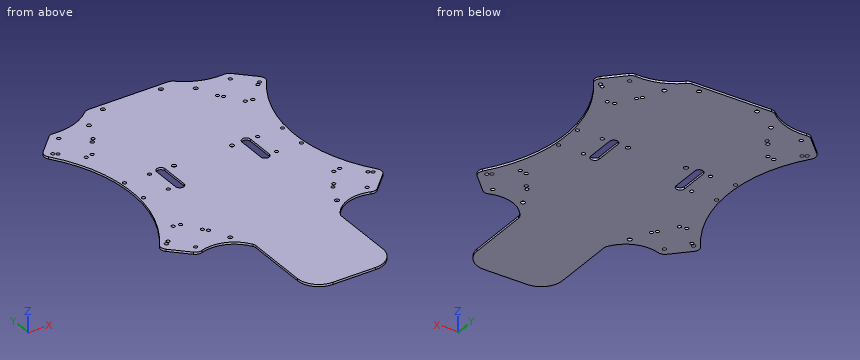
from build123d import *

# Parameters (mm, degrees)
SKETCH2_R           = 1.5
SKETCH2_R_2         = 1.25
BOSS_EXTRUDE1_DEPTH = 1.5
SKETCH3_R           = 1.25
F_45_DEGREES_DEPTH  = 170.629743854
SKETCH4_R           = 1.5
ODROID_HOLES_DEPTH  = 170.629743854
FILLET1_R           = 5
FILLET2_R           = 5
FILLET3_R           = 5
FILLET4_R           = 5
FILLET5_R           = 5
FILLET6_R           = 5
FILLET7_R           = 5
FILLET8_R           = 5
FILLET9_R           = 5
FILLET10_R          = 5
FILLET11_R          = 5
FILLET12_R          = 5
SKETCH5_R           = 1.25
F_35_DEGREES_DEPTH  = 169.878448293


with BuildPart() as part:
    # Sketch2 → Boss-Extrude1 (new body)
    with BuildSketch(Plane.XY):
        with BuildLine():
            Line((-79.195959493, 62.225396744), (-62.225396744, 79.195959493))
            ThreePointArc((-62.225396744, 79.195959493), (-44.806778225, 80.702789346), (-30, 90))
            Line((-30, 90), (30, 90))
            ThreePointArc((30, 90), (44.806778225, 80.702789346), (62.225396744, 79.195959493))
            Line((62.225396744, 79.195959493), (79.195959493, 62.225396744))
            ThreePointArc((79.195959493, 62.225396744), (57.477502656, 0), (79.195959493, -62.225396744))
            Line((79.195959493, -62.225396744), (62.225396744, -79.195959493))
            ThreePointArc((62.225396744, -79.195959493), (43.875108319, -77.923881554), (30, -90))
            Line((30, -90), (30, -135))
            ThreePointArc((30, -135), (25.606601718, -145.606601718), (15, -150))
            Line((15, -150), (-15, -150))
            ThreePointArc((-15, -150), (-25.606601718, -145.606601718), (-30, -135))
            Line((-30, -135), (-30, -90))
            ThreePointArc((-30, -90), (-43.875108319, -77.923881554), (-62.225396744, -79.195959493))
            Line((-62.225396744, -79.195959493), (-79.195959493, -62.225396744))
            ThreePointArc((-79.195959493, -62.225396744), (-57.477502656, 0), (-79.195959493, 62.225396744))
        make_face()
        with Locations((-37.5, 75)):
            Circle(SKETCH2_R, mode=Mode.SUBTRACT)
        with Locations((37.5, 75)):
            Circle(SKETCH2_R, mode=Mode.SUBTRACT)
        with Locations((37.5, -75)):
            Circle(SKETCH2_R, mode=Mode.SUBTRACT)
        with Locations((-37.5, -75)):
            Circle(SKETCH2_R, mode=Mode.SUBTRACT)
        with Locations((-55.5, 10)):
            Circle(SKETCH2_R_2, mode=Mode.SUBTRACT)
        with Locations((-38, 10)):
            Circle(SKETCH2_R_2, mode=Mode.SUBTRACT)
        with Locations((-55.5, -10)):
            Circle(SKETCH2_R_2, mode=Mode.SUBTRACT)
        with Locations((-38, -10)):
            Circle(SKETCH2_R_2, mode=Mode.SUBTRACT)
        with Locations((55.5, -10)):
            Circle(SKETCH2_R_2, mode=Mode.SUBTRACT)
        with Locations((38, -10)):
            Circle(SKETCH2_R_2, mode=Mode.SUBTRACT)
        with Locations((38, 10)):
            Circle(SKETCH2_R_2, mode=Mode.SUBTRACT)
        with Locations((55.5, 10)):
            Circle(SKETCH2_R_2, mode=Mode.SUBTRACT)
        with BuildLine():
            Line((27, -10), (27, 10))
            ThreePointArc((27, 10), (30, 13), (33, 10))
            Line((33, 10), (33, -10))
            ThreePointArc((33, -10), (30, -13), (27, -10))
        make_face(mode=Mode.SUBTRACT)
        with BuildLine():
            Line((-27, -10), (-27, 10))
            ThreePointArc((-27, 10), (-30, 13), (-33, 10))
            Line((-33, 10), (-33, -10))
            ThreePointArc((-33, -10), (-30, -13), (-27, -10))
        make_face(mode=Mode.SUBTRACT)
    extrude(amount=BOSS_EXTRUDE1_DEPTH)

    # Sketch3 → 45 Degrees (cut, through all)
    with BuildSketch(Plane.XY.offset(1.5)):
        with Locations((-72.655221767, 60.280853096)):
            Circle(SKETCH3_R)
        with Locations((-58.513086143, 46.138717472)):
            Circle(SKETCH3_R)
        with Locations(Location((-60.280853096, 72.655221767, 0), (0, 0, 180))):
            Circle(SKETCH3_R)
        with Locations(Location((-46.138717472, 58.513086143, 0), (0, 0, 180))):
            Circle(SKETCH3_R)
        with Locations(Location((58.513086143, 46.138717472, 0), (0, 0, 180))):
            Circle(SKETCH3_R)
        with Locations(Location((72.655221767, 60.280853096, 0), (0, 0, 180))):
            Circle(SKETCH3_R)
        with Locations((60.280853096, 72.655221767)):
            Circle(SKETCH3_R)
        with Locations((46.138717472, 58.513086143)):
            Circle(SKETCH3_R)
        with Locations(Location((-58.513086143, -46.138717472, 0), (0, 0, 180))):
            Circle(SKETCH3_R)
        with Locations((-46.138717472, -58.513086143)):
            Circle(SKETCH3_R)
        with Locations((-60.280853096, -72.655221767)):
            Circle(SKETCH3_R)
        with Locations(Location((-72.655221767, -60.280853096, 0), (0, 0, 180))):
            Circle(SKETCH3_R)
        with Locations((58.513086143, -46.138717472)):
            Circle(SKETCH3_R)
        with Locations((72.655221767, -60.280853096)):
            Circle(SKETCH3_R)
        with Locations(Location((60.280853096, -72.655221767, 0), (0, 0, 180))):
            Circle(SKETCH3_R)
        with Locations(Location((46.138717472, -58.513086143, 0), (0, 0, 180))):
            Circle(SKETCH3_R)
    extrude(amount=-F_45_DEGREES_DEPTH, mode=Mode.SUBTRACT)

    # Sketch4 → ODroid holes (cut, through all)
    with BuildSketch(Plane.XY.offset(1.5)):
        with Locations((-20.76, 10)):
            Circle(SKETCH4_R)
        with Locations((20, 10)):
            Circle(SKETCH4_R)
        with Locations((-20.76, 85.5)):
            Circle(SKETCH4_R)
        with Locations((20, 85.5)):
            Circle(SKETCH4_R)
    extrude(amount=-ODROID_HOLES_DEPTH, mode=Mode.SUBTRACT)

    # Fillet1
    fillet1_edges = [part.edges().sort_by_distance(p)[0] for p in [
        (-30, -90, 0.75),
    ]]
    fillet(fillet1_edges, radius=FILLET1_R)

    # Fillet2
    fillet2_edges = [part.edges().sort_by_distance(p)[0] for p in [
        (-62.225396744, -79.195959493, 0.75),
    ]]
    fillet(fillet2_edges, radius=FILLET2_R)

    # Fillet3
    fillet3_edges = [part.edges().sort_by_distance(p)[0] for p in [
        (30, -90, 0.75),
    ]]
    fillet(fillet3_edges, radius=FILLET3_R)

    # Fillet4
    fillet4_edges = [part.edges().sort_by_distance(p)[0] for p in [
        (62.225396744, -79.195959493, 0.75),
    ]]
    fillet(fillet4_edges, radius=FILLET4_R)

    # Fillet5
    fillet5_edges = [part.edges().sort_by_distance(p)[0] for p in [
        (79.195959493, -62.225396744, 0.75),
    ]]
    fillet(fillet5_edges, radius=FILLET5_R)

    # Fillet6
    fillet6_edges = [part.edges().sort_by_distance(p)[0] for p in [
        (-79.195959493, -62.225396744, 0.75),
    ]]
    fillet(fillet6_edges, radius=FILLET6_R)

    # Fillet7
    fillet7_edges = [part.edges().sort_by_distance(p)[0] for p in [
        (-79.195959493, 62.225396744, 0.75),
    ]]
    fillet(fillet7_edges, radius=FILLET7_R)

    # Fillet8
    fillet8_edges = [part.edges().sort_by_distance(p)[0] for p in [
        (-62.225396744, 79.195959493, 0.75),
    ]]
    fillet(fillet8_edges, radius=FILLET8_R)

    # Fillet9
    fillet9_edges = [part.edges().sort_by_distance(p)[0] for p in [
        (-30, 90, 0.75),
    ]]
    fillet(fillet9_edges, radius=FILLET9_R)

    # Fillet10
    fillet10_edges = [part.edges().sort_by_distance(p)[0] for p in [
        (30, 90, 0.75),
    ]]
    fillet(fillet10_edges, radius=FILLET10_R)

    # Fillet11
    fillet11_edges = [part.edges().sort_by_distance(p)[0] for p in [
        (62.225396744, 79.195959493, 0.75),
    ]]
    fillet(fillet11_edges, radius=FILLET11_R)

    # Fillet12
    fillet12_edges = [part.edges().sort_by_distance(p)[0] for p in [
        (79.195959493, 62.225396744, 0.75),
    ]]
    fillet(fillet12_edges, radius=FILLET12_R)

    # Sketch5 → 35 Degrees (cut, through all)
    with BuildSketch(Plane.XY.offset(1.5)):
        with Locations(Location((-60.280853096, 72.655221767, 0), (0, 0, 180))):
            Circle(SKETCH5_R)
        with Locations((-70.218840229, 58.462305252)):
            Circle(SKETCH5_R)
        with Locations((-53.835799344, 46.990776525)):
            Circle(SKETCH5_R)
        with Locations((-43.79882923, 61.326369694)):
            Circle(SKETCH5_R)
        with Locations((60.280853096, 72.655221767)):
            Circle(SKETCH5_R)
        with Locations(Location((43.79882923, 61.326369694, 0), (0, 0, 180))):
            Circle(SKETCH5_R)
        with Locations(Location((53.835799344, 46.990776525, 0), (0, 0, 180))):
            Circle(SKETCH5_R)
        with Locations(Location((70.218840229, 58.462305252, 0), (0, 0, 180))):
            Circle(SKETCH5_R)
        with Locations(Location((-70.218840229, -58.462305252, 0), (0, 0, 180))):
            Circle(SKETCH5_R)
        with Locations((-60.280853096, -72.655221767)):
            Circle(SKETCH5_R)
        with Locations(Location((-53.835799344, -46.990776525, 0), (0, 0, 180))):
            Circle(SKETCH5_R)
        with Locations(Location((-43.79882923, -61.326369694, 0), (0, 0, 180))):
            Circle(SKETCH5_R)
        with Locations((70.218840229, -58.462305252)):
            Circle(SKETCH5_R)
        with Locations(Location((60.280853096, -72.655221767, 0), (0, 0, 180))):
            Circle(SKETCH5_R)
        with Locations((43.79882923, -61.326369694)):
            Circle(SKETCH5_R)
        with Locations((53.835799344, -46.990776525)):
            Circle(SKETCH5_R)
    extrude(amount=-F_35_DEGREES_DEPTH, mode=Mode.SUBTRACT)


solid = part.part
Part model, mm, in its own coordinate system. Coordinates: 2 decimals unless noted, no trailing zeros. Loops run counter-clockwise (first coordinate to the right, second up) from the corner with the lowest first, then second, coordinate; pieces in that order, holes last. Notation, with made-up numbers: M 18.25,47 L 32.25,47 A16 ccw 32.25,65 Z; hole C 56.5,-29.5 d5. An arc over 180 degrees is marked long. Use a Markdown table: item, result. Add a question column.
Q1. Cut at B-B (z = 0.45). Give the number of separate pieces and of enclosed holes in the cut face, and give its area (3 significant figures).
Q2. Probe L1, parallel to Y at x = -70, z = 0.8; L2, parallel to Y at x = -46, z = 1.1; L3, parallel to X at y = -73, z = 0.9. List the from-to ranges inside material, lowest first.
Q3. Pin check, flat tips, straight feed: P1, Ø3, axis at x = 38, y = 10, coming from the -Z side; P2, Ø2.5, axis at x = 20, y = 10, coming from the -Z side; P3, Ø0.8, axis at y = 1.5, z = 1, coming from the -X side. Stop position of each tip, or through.
Q4. Cut at A-A (y = -108). Write the cut outline in (x, z), and give its area (3 significant figures).
Worked out:
| question | item | result |
|---|---|---|
| 1 | separate pieces | 1 |
| 1 | enclosed holes | 46 |
| 1 | area | 25,200 mm2 |
| 2 | L1 | y = -71.42 to -59.69, -57.23 to -48.45, 48.45 to 57.23, 59.69 to 71.42 |
| 2 | L2 | y = -77.32 to -59.76, -57.27 to 57.27, 59.76 to 80.32 |
| 2 | L3 | x = -68.42 to -61.48, -59.08 to 59.08, 61.48 to 68.42 |
| 3 | P1 | stops at z = 0 |
| 3 | P2 | passes through |
| 3 | P3 | stops at x = -57.5 |
| 4 | outline | M -30,0 L 30,0 L 30,1.5 L -30,1.5 Z |
| 4 | area | 90.0 mm2 |
